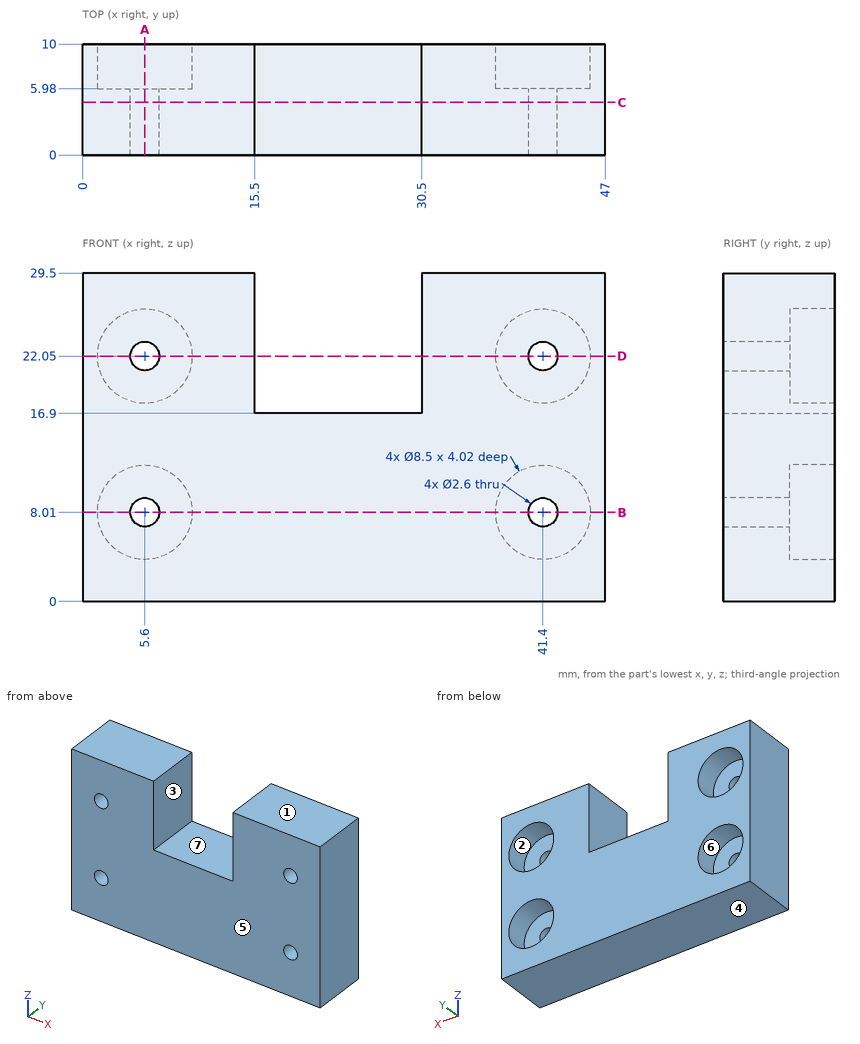
For this review, use the dimensioned drawing (mm, ordinates from the lowest corner) and the shaded views. A direction names the side the tool comes from. Give positions to 0.01 mm unless a question says otherwise; leave off trailing zeros. Write each loop counter-clockwise with the first axis right and the second up, starting at its lowest first coordinate (ties: lowest second). Pieces come first, ordered by that corner, then holes. Notation, with made-up numbers: M 66,-5 L 90,-5 A35 cw 90,31 Z; hole C 65.25,27 d6. An arc over 180 degrees is marked long. Answer as a JSON object with one key per item and string values. Group by question number.
1) We need section A-A (x = 5.6). Give the boundary of the cut face in (y, z), and give its area (3 significant figures).
2) Mouldability with a two-part tool opening along Z and no side actions: class the marked faces 1, 2, 3 and 4 as released by +Z, released by -Z, zero draft, split by the parting line, or undercut.
3) For line 1 along X through (y, z) = (1.6, 22.05); line 2 along X through (y, z) = (7.1, 8.01); line 3 along Z through (x, y) = (8, 8), list the stretches that pass through material, from the lowest coordinate up.
4) We need section C-C (y = 4.75). Give the boundary of the cut face in (x, z), and give its area (3 significant figures).
5) We need section B-B (z = 8.01). Give the boundary of the cut face in (x, y).
6) We need section D-D (z = 22.05). Give the boundary of the cut face in (x, y).
7) Tool access review of the marked faces 5, 6 and 7: name each direction out of +Z, -Z, +X, -X, +Y, -Y from which nothing blocks a thin tool from reaching the whole face with its end or side.
8) Clearance check with flat-ended pins moving along their axes: pin 1 Ø7.5 at (x, z) = (5.6, 22.05) entering from +Y; pin 2 Ø2 at (x, z) = (41.4, 8.01) entering from +Y. State where each tip first meets the part, or that it passes through.
Answer key:
{
 "1": {"outline": "M 0,0 L 10,0 L 10,3.76 L 5.98,3.76 L 5.98,6.71 L 0,6.71 Z; M 0,9.31 L 5.98,9.31 L 5.98,12.26 L 10,12.26 L 10,17.8 L 5.98,17.8 L 5.98,20.75 L 0,20.75 Z; M 0,23.35 L 5.98,23.35 L 5.98,26.3 L 10,26.3 L 10,29.5 L 0,29.5 Z", "area": "196 mm²"},
 "2": {"face 1": "released by +Z", "face 2": "undercut", "face 3": "zero draft", "face 4": "released by -Z"},
 "3": {"line 1": "x = 0 to 4.3, 6.9 to 15.5, 30.5 to 40.1, 42.7 to 47", "line 2": "x = 0 to 1.35, 9.85 to 37.15, 45.65 to 47", "line 3": "z = 0 to 4.5, 11.52 to 18.54, 25.56 to 29.5"},
 "4": {"outline": "M 0,0 L 47,0 L 47,29.5 L 30.5,29.5 L 30.5,16.9 L 15.5,16.9 L 15.5,29.5 L 0,29.5 Z; hole C 5.6,8.01 d2.6; hole C 5.6,22.05 d2.6; hole C 41.4,8.01 d2.6; hole C 41.4,22.05 d2.6", "area": "1,180 mm²"},
 "5": {"outline": "M 0,0 L 4.3,0 L 4.3,5.98 L 1.35,5.98 L 1.35,10 L 0,10 Z; M 6.9,0 L 40.1,0 L 40.1,5.98 L 37.15,5.98 L 37.15,10 L 9.85,10 L 9.85,5.98 L 6.9,5.98 Z; M 42.7,0 L 47,0 L 47,10 L 45.65,10 L 45.65,5.98 L 42.7,5.98 Z"},
 "6": {"outline": "M 0,0 L 4.3,0 L 4.3,5.98 L 1.35,5.98 L 1.35,10 L 0,10 Z; M 6.9,0 L 15.5,0 L 15.5,10 L 9.85,10 L 9.85,5.98 L 6.9,5.98 Z; M 30.5,0 L 40.1,0 L 40.1,5.98 L 37.15,5.98 L 37.15,10 L 30.5,10 Z; M 42.7,0 L 47,0 L 47,10 L 45.65,10 L 45.65,5.98 L 42.7,5.98 Z"},
 "7": {"face 5": "+Z, -Z, +X, -X, -Y", "face 6": "+Y", "face 7": "+Z, +Y, -Y"},
 "8": {"pin 1": "stops at y = 5.98", "pin 2": "passes through"}
}
